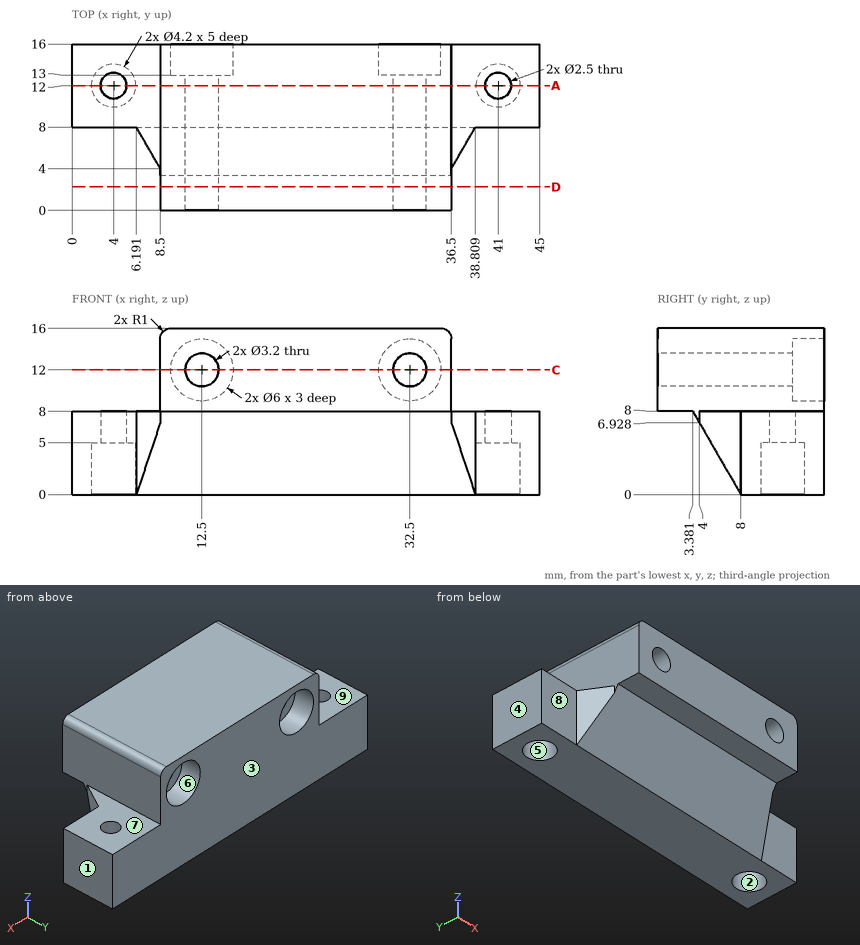
Drawing for the job (mm, zero at the part's lowest x, y, z). A direction names the side the tool comes from. Round coordinates to 2 decimals unless told otherwise and drop trailing zeros. Write each loop counter-clockwise with the first axis right and the second up, starting at its lowest first coordinate (ties: lowest second). Pieces come first, ordered by that corner, then holes. Notation, with made-up numbers: M -40,33 L -4,33 A17 ccw -4,52 Z; hole C -27,36 d7. An arc over 180 degrees is marked long. Put each result on its own line as item: value.
Item 1: Cut at D-D (y = 2.25). List the corners of the cut face in (x, z).
Responses:
outline: M 8.5,8 L 36.5,8 L 36.5,15 A1 ccw 35.5,16 L 9.5,16 A1 ccw 8.5,15 Z; hole C 12.5,12 d3.2; hole C 32.5,12 d3.2
Item 2: Cut at C-C (z = 12). List the corners of the cut face in (x, y), and give its area (3 significant figures).
Responses:
outline: M 8.5,0 L 10.9,0 L 10.9,13 L 9.5,13 L 9.5,16 L 8.5,16 Z; M 14.1,0 L 30.9,0 L 30.9,13 L 29.5,13 L 29.5,16 L 15.5,16 L 15.5,13 L 14.1,13 Z; M 34.1,0 L 36.5,0 L 36.5,16 L 35.5,16 L 35.5,13 L 34.1,13 Z
area: 329 mm²
Item 3: Cut at A-A (y = 12). List the corners of the cut face in (x, z).
Responses:
outline: M 0,0 L 1.9,0 L 1.9,5 L 2.75,5 L 2.75,8 L 0,8 Z; M 5.25,5 L 6.1,5 L 6.1,0 L 38.9,0 L 38.9,5 L 39.75,5 L 39.75,8 L 36.5,8 L 36.5,15 A1 ccw 35.5,16 L 9.5,16 A1 ccw 8.5,15 L 8.5,8 L 5.25,8 Z; M 42.25,5 L 43.1,5 L 43.1,0 L 45,0 L 45,8 L 42.25,8 Z; hole C 12.5,12 d3.2; hole C 32.5,12 d3.2
Item 4: Tool access for the marked faces 5, 6, 7, 8 and 9: list every direction of +Z, -Z, +X, -X, +Y, -Y with a clear straight run to the whole face (end or side of a thin tool).
Responses:
face 5: -Z
face 6: +Y
face 7: +Z, +X, +Y, -Y
face 8: +Z, -Z, -X, -Y
face 9: +Z, -X, +Y, -Y
Item 5: Mould opens along X. For the marked faces 1, 2, 3 and 4 say: +X half, -X half, draft (parallel to the pull), parting line (faces both ways), or undercut.
Responses:
face 1: +X half
face 2: undercut
face 3: draft
face 4: -X half
Item 6: Probe L1, parallel to X at y = 14.55, z = 12; L2, parallel to X at y = 10.5, z = 12; L3, parallel to Z at x = 2.5, y = 9. List the from-to ranges inside material, lowest first. Write a range as from..to.
Responses:
L1: 8.5..9.5, 15.5..29.5, 35.5..36.5
L2: 8.5..10.9, 14.1..30.9, 34.1..36.5
L3: 0..8
Item 7: Flat gauge pins, fed straight in: P1, Ø5.5, axis at x = 41, y = 12, coming from the +Z side; P2, Ø1, axis at y = 5, z = 12.5, coming from the +X side; P3, Ø4, axis at x = 41, y = 12, coming from the -Z side. Where does each tip first touch, or does it go through?
Responses:
P1: z = 8
P2: x = 36.5
P3: z = 5
